Read the model definition and answer for the solid it produces. Units are mm, in the model's axes. A direction names the side the tool comes from. Coordinates: 2 decimals unless noted, no trailing zeros. Write each loop counter-clockwise with the first axis right and the second up, starting at its lowest first coordinate (ties: lowest second). Pieces come first, ordered by that corner, then holes. Notation, with made-up numbers: (-18.75, 38.5) -> (29.25, 38.5) arc R23 ccw to (29.25, 46.5) -> close; hole circle Ø9 at (4, 45). An arc over 180 degrees is marked (long way). Answer in a Markdown table with one row per item. Add a question column.
Item 1: Section C-C on x = 5 is taken. Write down the section's boundary in (y, z) (3 decimals).
Item 2: Section B-B on z = -7.5 is taken. Write down the section's boundary in (x, y) (3 decimals).
Item 3: Section D-D on z = -51.5 is taken. Write down the section's boundary in (x, y).
Item 4: Which of the six approach directions +Z, -Z, +X, -X, +Y, -Y give full straight-line access (tool end or side, diameter ignored) to faces 1 (the face through (5, 2, -64)), 2 (the face through (5, 27, -79)), 3 (the face through (5, 6, -3))?
Item 5: Section A-A on y = 15.5 is taken. Write down the section's boundary in (x, z).
Item 6: Straight lines are drawn through the part: line 1 (Z direction, x = 5, y = 2.4); line 2 (Z direction, x = 2.5, y = 39.5); line 3 (Y direction, x = 9.5, z = -8.5). For each, find the intervals that lie inside material, in ascending order. Write a range as from..to.
Item 7: Given pin 1 Ø5 at (x, z) = (6, -48) entering from -Y, flat-ended and moving along its own axis, determine where the tip first touches the part or whether it passes through.
Autodesk Fusion 360 part; units mm, degrees
sketch "Sketch1" plane through (0, 0, 0) normal (1, 0, 0) x (0, 0, -1)
  line L0 (0, 0) -> (15, 0)
  line L1 (15, 0) -> (15, 4)
  line L2 (15, 4) -> (3, 4)
  line L3 (3, 4) -> (3, 8.4)
  line L4 (3, 8.4) -> (6, 8.4)
  line L5 (6, 8.4) -> (6, 50)
  line L6 (6, 50) -> (39.5, 50)
  line L7 (39.5, 54) -> (0, 54)
  line L8 (0, 54) -> (0, 0)
  line L9 (39.5, 54) -> (39.5, 50) construction
  line L10 (64, 0) -> (64, 4)
  line L11 (79, 0) -> (64, 0)
  line L12 (73, 8.4) -> (73, 50)
  line L13 (76, 4) -> (76, 8.4)
  line L14 (76, 8.4) -> (73, 8.4)
  line L15 (79, 54) -> (79, 0)
  line L16 (64, 4) -> (76, 4)
  line L17 (73, 50) -> (39.5, 50)
  line L18 (39.5, 54) -> (79, 54)
  point P0 (79, 0)
  dimension "d1" = 4.4
  dimension "d3" = 6
  dimension "d4" = 4
  dimension "d5" = 50
  dimension "d7" = 73
  dimension "d8" = 4
  dimension "d11" = 3
  dimension "d12" = 15
extrude "Extrude1" add sketch "Sketch1" along normal blind 10
ref_plane "WorkPlane1" through (5, 27, -39.5) normal (0, 0, -1) x (0, 1, 0)
hole "Hole2" at (5, 0, -7.5) direction (0, 1, 0) diameter 4.5 depth 5 tip angle 118 countersink diameter 4.95 countersink angle 90
mirror "Mirror1" about plane through (5, 27, -39.5) normal (0, 0, -1) of "Hole2"
Results below:
| question | item | result |
|---|---|---|
| 1 | outline | (0, -79) -> (54, -79) -> (54, 0) -> (0, 0) -> (0, -5.025) -> (0.225, -5.25) -> (4, -5.25) -> (4, -3) -> (8.4, -3) -> (8.4, -6) -> (50, -6) -> (50, -73) -> (8.4, -73) -> (8.4, -76) -> (4, -76) -> (4, -73.75) -> (0.225, -73.75) -> (0, -73.975) -> close; (0, -69.025) -> (0.225, -69.25) -> (4, -69.25) -> (4, -64) -> (0, -64) -> close; (0, -15) -> (4, -15) -> (4, -9.75) -> (0.225, -9.75) -> (0, -9.975) -> close |
| 2 | outline | (0, 0) -> (2.525, 0) -> (2.75, 0.225) -> (2.75, 4) -> (0, 4) -> close; (0, 50) -> (10, 50) -> (10, 54) -> (0, 54) -> close; (7.25, 0.225) -> (7.475, 0) -> (10, 0) -> (10, 4) -> (7.25, 4) -> close |
| 3 | outline | (0, 50) -> (10, 50) -> (10, 54) -> (0, 54) -> close |
| 4 | face 1 | +X, -X, -Y |
| 4 | face 2 | -Z, +X, -X, +Y, -Y |
| 4 | face 3 | +X, -X |
| 5 | outline | (0, -79) -> (10, -79) -> (10, -73) -> (0, -73) -> close; (0, -6) -> (10, -6) -> (10, 0) -> (0, 0) -> close |
| 6 | line 1 | z = -79..-73.75, -69.25..-64, -15..-9.75, -5.25..0 |
| 6 | line 2 | z = -79..-73, -6..0 |
| 6 | line 3 | y = 0..4, 50..54 |
| 7 | pin 1 | stops at y = 50 |
